```python
from build123d import *

# Parameters (mm, degrees)
SKETCH_1_R      = 1.5
SKETCH_1_W      = 10
SKETCH_1_H      = 3
EXTRUDE_1_DEPTH = 3
FILLET_1_R      = 10


with BuildPart() as part:
    # 草图1 → 凸台-拉伸1 (new body)
    with BuildSketch(Plane(origin=(0, 0, 0), x_dir=(1, 0, 0), z_dir=(0, 1, 0))):
        with BuildLine():
            Line((-55.885621722, -7.5), (55.885621722, -7.5))
            ThreePointArc((55.885621722, -7.5), (72.5, 0), (55.885621722, 7.5))
            Line((55.885621722, 7.5), (-55.885621722, 7.5))
            ThreePointArc((-55.885621722, 7.5), (-72.5, 0), (-55.885621722, -7.5))
        make_face()
        with Locations(Location((-62.5, 0, 0), (0, 0, 270))):
            Circle(SKETCH_1_R, mode=Mode.SUBTRACT)
        with Locations(Location((62.5, 0, 0), (0, 0, 270))):
            Circle(SKETCH_1_R, mode=Mode.SUBTRACT)
        with Locations((-15, 0)):
            Rectangle(SKETCH_1_W, SKETCH_1_H, mode=Mode.SUBTRACT)
        with Locations((15, -0.064058726)):
            Rectangle(SKETCH_1_W, SKETCH_1_H, mode=Mode.SUBTRACT)
    extrude(amount=EXTRUDE_1_DEPTH)

    # 圆角1
    fillet_1_edges = [part.edges().sort_by_distance(p)[0] for p in [
        (-55.885621722, 1.5, -7.5),
        (55.885621722, 1.5, -7.5),
        (55.885621722, 1.5, 7.5),
        (-55.885621722, 1.5, 7.5),
    ]]
    fillet(fillet_1_edges, radius=FILLET_1_R)


solid = part.part
```
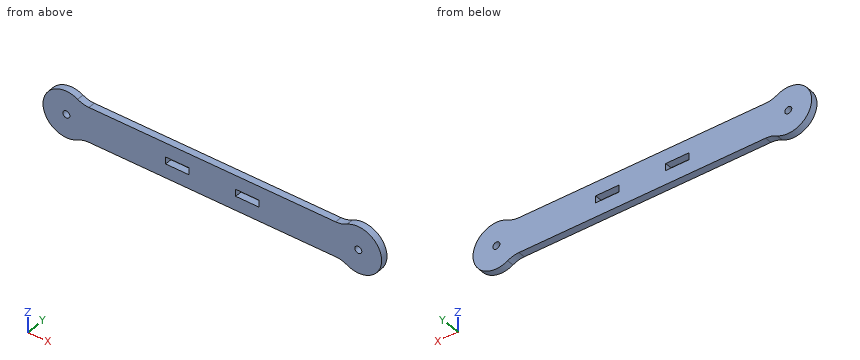
Design review of the part built by this model. Coordinates are the model's own, in mm. Coordinates: 2 decimals unless noted, no trailing zeros. Order: outer loops, then holes, each group sorted by start corner. A loop starts at its lowest first (then second) coordinate and runs counter-clockwise, first axis right, second up. Notation, with made-up numbers: (-10, 23.25) - (46, 23.25) arc R9 ccw to (46, 28.25) - close; hole circle Ø11 at (-26.75, -29). An arc over 180 degrees is marked (long way). Answer in a Markdown table with one row per item.
(1) Clearance check with flat-ended pins moving along their axes: pin 1 (1.5 mm diameter, centred on y = 1.5, z = 0.5, fed in from -X); pin 2 (1.5 mm diameter, centred on x = -13, y = 1.5, fed in from -Z); pin 3 (2.5 mm diameter, centred on x = 62.5, z = 0, fed in from -Y). State where each tip first meets the part, or that it passes through.
Checked values:
| item | result |
|---|---|
| pin 1 | x = -72.5 |
| pin 2 | z = -7.5 |
| pin 3 | through |
(2) Wall thickness on line 1 along Z through (x, y) = (19.5, 0.95); line 2 along X through (y, z) = (1.5, 0); line 3 along Z through (x, y) = (50.5, 0.3): over which ranges is each line inside the solid? List them lowest first. Write a range as from..to.
Checked values:
| item | result |
|---|---|
| line 1 | -7.5..-1.44, 1.56..7.5 |
| line 2 | -72.5..-64, -61..-20, -10..10, 20..61, 64..72.5 |
| line 3 | -7.5..7.5 |
(3) Consider section B-B on y = 1.25. State the section outline as (x, z) points.
Checked values:
| item | result |
|---|---|
| outline | (-57.66, -8.75) arc R10 cw to (-52.82, -7.5) - (52.82, -7.5) arc R10 cw to (57.66, -8.75) arc R10 ccw (long way) to (57.66, 8.75) arc R10 cw to (52.82, 7.5) - (-52.82, 7.5) arc R10 cw to (-57.66, 8.75) arc R10 ccw (long way) to start; hole circle Ø3 at (-62.5, 0); hole (-20, -1.5) - (-10, -1.5) - (-10, 1.5) - (-20, 1.5) - close; hole (10, -1.44) - (20, -1.44) - (20, 1.56) - (10, 1.56) - close; hole circle Ø3 at (62.5, 0) |
(4) Consider section D-D on x = -6. State the section outline as (y, z) points, plus the area to 3 significant figures.
Checked values:
| item | result |
|---|---|
| outline | (0, -7.5) - (3, -7.5) - (3, 7.5) - (0, 7.5) - close |
| area | 45.0 mm^2 |
(5) Consider section A-A on x = -62.5. State the section outline as (y, z) points, plus the area to 3 significant figures.
Checked values:
| item | result |
|---|---|
| outline | (0, -10) - (3, -10) - (3, -1.5) - (0, -1.5) - close; (0, 1.5) - (3, 1.5) - (3, 10) - (0, 10) - close |
| area | 51.0 mm^2 |
(6) Consider section C-C on x = 17.5. State the section outline as (y, z) points.
Checked values:
| item | result |
|---|---|
| outline | (0, -7.5) - (3, -7.5) - (3, -1.44) - (0, -1.44) - close; (0, 1.56) - (3, 1.56) - (3, 7.5) - (0, 7.5) - close |
